```python
from build123d import *

# Parameters (mm, degrees)
F0_W         = 30
F0_H         = 30
F1_DEPTH     = 15
F2_W         = 9.8
F2_H         = 9.8
F3_DEPTH     = 10
F4_W         = 10.2
F4_H         = 10.2
F5_DEPTH     = 21
F6_W         = 10.2
F6_H         = 10.2
F7_DEPTH     = 30
F8_W         = 10.2
F8_H         = 10.2
F9_DEPTH     = 30.001
F10_T1_DEPTH = 20.9121426428
F10_T3_DEPTH = 20.9121426428


# Not quite as in the source:
# - a fillet or chamfer that OpenCascade refuses, or shapes differently, is made with other operations: its cross-section is extruded or revolved along the edge and cut away or added


with BuildPart() as f1:
    # F0 (on Front) → F1 (new body, symmetric)
    with BuildSketch(Plane.XZ):
        Rectangle(F0_W, F0_H)
    extrude(amount=F1_DEPTH, both=True)

    # F2 (on face) → F3 (join)
    with BuildSketch(Plane.XY.offset(15)):
        Rectangle(F2_W, F2_H)
    extrude(amount=F3_DEPTH)

    # F4 (on face) → F5 (cut)
    with BuildSketch(Plane(origin=(0, 0, -15), x_dir=(1, 0, 0), z_dir=(0, 0, -1))):
        Rectangle(F4_W, F4_H)
    extrude(amount=-F5_DEPTH, mode=Mode.SUBTRACT)

    # F6 (on face) → F7 (cut)
    with BuildSketch(Plane.YZ.offset(15)):
        Rectangle(F6_W, F6_H)
    extrude(amount=-F7_DEPTH, mode=Mode.SUBTRACT)

    # F8 (on face) → F9 (cut, through all)
    with BuildSketch(Plane.XZ.offset(15)):
        Rectangle(F8_W, F8_H)
    extrude(amount=-F9_DEPTH, mode=Mode.SUBTRACT)

    # F10: fillet of radius 3 on 4 edges, made by hand

    # F10_s2 → F10_t1 (join)
    with BuildSketch(Plane.YZ.offset(-10.4560713214)):
        with BuildLine():
            ThreePointArc((-5.1, 5.1), (-4.1194664753, 5.7658633372), (-2.9575714714, 6))
            Line((-2.9575714714, 6), (-5.1, 6))
            Line((-5.1, 6), (-5.1, 5.1))
        make_face()
        with BuildLine():
            ThreePointArc((5.1, 5.1), (4.1194664753, 5.7658633372), (2.9575714714, 6))
            Line((2.9575714714, 6), (5.1, 6))
            Line((5.1, 6), (5.1, 5.1))
        make_face()
    extrude(amount=F10_T1_DEPTH)

    # F10_s4 → F10_t3 (join)
    with BuildSketch(Plane.XZ.offset(-10.4560713214)):
        with BuildLine():
            ThreePointArc((5.1, 5.1), (4.1194664753, 5.7658633372), (2.9575714714, 6))
            Line((2.9575714714, 6), (5.1, 6))
            Line((5.1, 6), (5.1, 5.1))
        make_face()
        with BuildLine():
            ThreePointArc((-2.9575714714, 6), (-4.1194664753, 5.7658633372), (-5.1, 5.1))
            Line((-5.1, 5.1), (-5.1, 6))
            Line((-5.1, 6), (-2.9575714714, 6))
        make_face()
    extrude(amount=F10_T3_DEPTH)


solid = f1.part
```
Source: CAD feature listing. Evaluate the final solid. Frame: model axes, mm. A direction names the side the tool comes from. Round coordinates to 2 decimals unless told otherwise and drop trailing zeros. Loops run counter-clockwise (first coordinate to the right, second up) from the corner with the lowest first, then second, coordinate; pieces in that order, holes last. Notation, with made-up numbers: M -17.75,25.25 L 31.25,25.25 A17 ccw 31.25,48.25 Z; hole C 55,-37 d10. An arc over 180 degrees is marked long. Use a Markdown table: item, result. Add a question column.
1. Mould query, pull axis Z, two halves, no side actions, for faces 1 (the flat face through (-5.1, -10, 0)), 2 (the cylindrical face through (-0.07, 4.13, 5.76)), 3 (the flat face through (0, 10, 5.1)), 4 (the flat face through (5.1, 0, -10)). Classes: pulls with the +Z half, pulls with the -Z half, needs draft (parallel to the pull), parting line crosses it, or undercut.
2. Section query A-A on y = 8.25. Return the cut outline in (x, z), then the cut area to 3 significant figures.
3. Section query B-B on z = 3.5. Return the cut outline in (x, y).
4. Section query C-C on x = -1. Return the cut outline in (y, z), then the cut area to 3 significant figures.
5. Contact query for flat-ended pins moving along their axis: P1, Ø2, axis at x = -5, y = -10.5, coming from the +Z side; P2, Ø3, axis at y = 0, z = 18, coming from the +X side. Output: stop coordinate, or through.
6. Line query: line 1 (Z direction, x = 0.25, y = -12). Output: solid intervals per line, ascending.
7. Reachability of faces 5 (the flat face through (5.1, 10, 0)), 6 (the flat face through (-4.9, 0, 20)), 7 (the flat face through (-5.1, 0, -10)) from +Z, -Z, +X, -X, +Y, -Y: full face, straight path, thin tool, end or side. Return the list, or none.
Reported:
| question | item | result |
|---|---|---|
| 1 | face 1 | undercut |
| 1 | face 2 | pulls with the -Z half |
| 1 | face 3 | undercut |
| 1 | face 4 | needs draft |
| 2 | outline | M -15,-15 L 15,-15 L 15,15 L -15,15 Z; hole M -5.1,-5.1 L 5.1,-5.1 L 5.1,5.1 L -5.1,5.1 Z |
| 2 | area | 796 mm² |
| 3 | outline | M -15,-15 L -5.1,-15 L -5.1,-5.1 L -15,-5.1 Z; M -15,5.1 L -5.1,5.1 L -5.1,15 L -15,15 Z; M 5.1,-15 L 15,-15 L 15,-5.1 L 5.1,-5.1 Z; M 5.1,5.1 L 15,5.1 L 15,15 L 5.1,15 Z |
| 4 | outline | M -15,-15 L -5.1,-15 L -5.1,-5.1 L -15,-5.1 Z; M -15,5.1 L -5.1,5.1 A3 cw -2.96,6 L 2.96,6 A3 cw 5.1,5.1 L 15,5.1 L 15,15 L 4.9,15 L 4.9,25 L -4.9,25 L -4.9,15 L -15,15 Z; M 5.1,-15 L 15,-15 L 15,-5.1 L 5.1,-5.1 Z |
| 4 | area | 583 mm² |
| 5 | P1 | stops at z = 15 |
| 5 | P2 | stops at x = 4.9 |
| 6 | line 1 | z = -15 to -5.1, 5.1 to 15 |
| 7 | face 5 | +Y, -Y |
| 7 | face 6 | +Z, -X, +Y, -Y |
| 7 | face 7 | -Z |
